The model under review builds one solid part; all positions refer to its coordinate system, in mm. Give positions to 0.01 mm unless a question says otherwise; leave off trailing zeros. Loops run counter-clockwise (first coordinate to the right, second up) from the corner with the lowest first, then second, coordinate; pieces in that order, holes last. Notation, with made-up numbers: (38.25, 88) - (88.25, 88) arc R11 cw to (88.25, 92) - close; hole circle Ø1 at (42.5, 48). An arc over 180 degrees is marked (long way). Answer as a JSON object with one key per item and string values.
from build123d import *

# Parameters (mm, degrees)
F0_R     = 2
F1_DEPTH = 9
F3_DEPTH = 9.001


with BuildPart() as f1:
    # F0 (on Front) → F1 (new body)
    with BuildSketch(Plane.XZ):
        Polygon((265.897079, -111.097285), (265.897079, 120.763555), (212.761675, 120.763555), (212.761675, 198.045397), (174.114259, 198.045397), (174.114259, 246.352586), (82.3411, 246.352586), (82.3411, 285.000002), (-130.196029, 285.000002), (-130.196029, 246.352586), (-217.152296, 246.352586), (-217.152296, 198.045397), (-265.461152, 198.045397), (-265.461152, 120.763555), (-182.215667, 120.657777), (-182.292131, 78.99439), (-40.622253, 80.756165), (-39.717878, 37.151925), (50.208882, 36.247385), (51.121586, -25.518982), (-39.717878, -26.429854), (-39.717878, -70.935305), (-180.510698, -71.846343), (-180.510698, -115.447249), (-265.897079, -116.364784), (-265.461152, -183.560564), (-217.152296, -183.560564), (-217.152296, -246.360741), (-130.196029, -246.360741), (-130.196029, -284.999998), (82.3411, -284.999998), (82.3411, -246.360741), (174.114259, -246.360741), (174.114259, -183.560564), (212.761675, -183.560564), (212.761675, -111.097285), align=None)
        with Locations((-169.174156, -241.860734)):
            Circle(F0_R, mode=Mode.SUBTRACT)
        with Locations((-236.821267, -179.060557)):
            Circle(F0_R, mode=Mode.SUBTRACT)
        with Locations((-212.652289, -210.460646)):
            Circle(F0_R, mode=Mode.SUBTRACT)
        with Locations((-261.179171, -149.93847)):
            Circle(F0_R, mode=Mode.SUBTRACT)
        with Locations((-125.696022, -261.180363)):
            Circle(F0_R, mode=Mode.SUBTRACT)
        with Locations((-23.927464, -280.499991)):
            Circle(F0_R, mode=Mode.SUBTRACT)
        with Locations((-218.689395, -120.357772)):
            Circle(F0_R, mode=Mode.SUBTRACT)
        with Locations((-176.010692, -98.108243)):
            Circle(F0_R, mode=Mode.SUBTRACT)
        with Locations((-105.614282, -75.861807)):
            Circle(F0_R, mode=Mode.SUBTRACT)
        with Locations((-35.217872, -53.145626)):
            Circle(F0_R, mode=Mode.SUBTRACT)
        with Locations((77.841094, -261.180363)):
            Circle(F0_R, mode=Mode.SUBTRACT)
        with Locations((123.727673, -241.860734)):
            Circle(F0_R, mode=Mode.SUBTRACT)
        with Locations((169.614252, -210.460646)):
            Circle(F0_R, mode=Mode.SUBTRACT)
        with Locations((188.937961, -179.060557)):
            Circle(F0_R, mode=Mode.SUBTRACT)
        with Locations((208.261669, -142.828918)):
            Circle(F0_R, mode=Mode.SUBTRACT)
        with Locations((10.235017, -30.429196)):
            Circle(F0_R, mode=Mode.SUBTRACT)
        with Locations((234.829371, -106.597278)):
            Circle(F0_R, mode=Mode.SUBTRACT)
        with Locations((-219.334275, 125.204953)):
            Circle(F0_R, mode=Mode.SUBTRACT)
        with Locations((-177.74558, 104.351434)):
            Circle(F0_R, mode=Mode.SUBTRACT)
        with Locations((-35.762538, 63.459567)):
            Circle(F0_R, mode=Mode.SUBTRACT)
        with Locations((-106.999755, 84.431064)):
            Circle(F0_R, mode=Mode.SUBTRACT)
        with Locations((-260.961145, 159.401619)):
            Circle(F0_R, mode=Mode.SUBTRACT)
        with Locations((-236.806717, 193.54539)):
            Circle(F0_R, mode=Mode.SUBTRACT)
        with Locations((-212.652289, 217.698985)):
            Circle(F0_R, mode=Mode.SUBTRACT)
        with Locations((-169.174156, 241.852579)):
            Circle(F0_R, mode=Mode.SUBTRACT)
        with Locations((-125.696022, 261.176288)):
            Circle(F0_R, mode=Mode.SUBTRACT)
        with Locations((-23.927464, 280.499996)):
            Circle(F0_R, mode=Mode.SUBTRACT)
        with Locations((55.165724, 5.364793)):
            Circle(F0_R, mode=Mode.SUBTRACT)
        with Locations((9.66711, 41.155414)):
            Circle(F0_R, mode=Mode.SUBTRACT)
        with Locations((261.397073, 4.833135)):
            Circle(F0_R, mode=Mode.SUBTRACT)
        with Locations((234.829371, 116.263548)):
            Circle(F0_R, mode=Mode.SUBTRACT)
        with Locations((123.727673, 241.852579)):
            Circle(F0_R, mode=Mode.SUBTRACT)
        with Locations((77.841094, 261.176288)):
            Circle(F0_R, mode=Mode.SUBTRACT)
        with Locations((188.937961, 193.54539)):
            Circle(F0_R, mode=Mode.SUBTRACT)
        with Locations((208.261669, 154.904469)):
            Circle(F0_R, mode=Mode.SUBTRACT)
        with Locations((169.614252, 217.698985)):
            Circle(F0_R, mode=Mode.SUBTRACT)
    extrude(amount=F1_DEPTH)

    # F2 (on face) → F3 (cut, through all)
    with BuildSketch(Plane(origin=(0, 0, 0), x_dir=(-1, 0, 0), z_dir=(0, 1, 0))):
        Polygon((-62.341114, 265.000015), (-62.341114, 226.352599), (-154.114272, 226.352599), (-154.114272, 178.04541), (-192.761689, 178.04541), (-192.761689, 100.763568), (-245.897092, 100.763568), (-245.897092, -91.097298), (-192.761689, -91.097298), (-192.761689, -163.560577), (-154.114272, -163.560577), (-154.114272, -226.360754), (-62.341114, -226.360754), (-62.341114, -265.000011), (110.196042, -265.000011), (110.196042, -226.360754), (197.152309, -226.360754), (197.152309, -163.560577), (245.590493, -163.560577), (245.768319, -136.149628), (160.510711, -135.233477), (160.510711, -91.717333), (19.717892, -90.806296), (19.717892, -46.230301), (-71.416299, -45.316474), (-69.918433, 56.050133), (20.124334, 56.95584), (21.037859, 101.001245), (162.254945, 99.245101), (162.178988, 140.63232), (245.461165, 140.738145), (245.461165, 178.04541), (197.152309, 178.04541), (197.152309, 226.352599), (110.196042, 226.352599), (110.196042, 265.000015), align=None)
    extrude(amount=-F3_DEPTH, mode=Mode.SUBTRACT)


solid = f1.part
Q1. To check wall thickness, follow probe 1 along X at (y, z) = (-6, 261.5); probe 2 along X at (y, z) = (-0.5, 166); probe 3 along X at (y, z) = (-1.75, -131). State the ranges of each line that lie inside material, in increasing order. Write a range as [from, to].
Results:
{"probe 1": "x = [-130.2, -127.67], [-123.72, -110.2], [62.34, 75.87], [79.81, 82.34]", "probe 2": "x = [-265.46, -245.46], [192.76, 212.76]", "probe 3": "x = [-265.8, -160.51], [192.76, 212.76]"}
Q2. Consider section A-A, the plane x = -79.5. State the section outline as (y, z) points.
Results:
{"outline": "(-9, -285) - (0, -285) - (0, -265) - (-9, -265) - close; (-9, -91.19) - (0, -91.19) - (0, -71.19) - (-9, -71.19) - close; (-9, 80.27) - (0, 80.27) - (0, 100.27) - (-9, 100.27) - close; (-9, 265) - (0, 265) - (0, 285) - (-9, 285) - close"}
Q3. Clearance check with flat-ended pins moving along their axes: pin 1 Ø4.5 at (x, y) = (-172.5, -5.5) entering from -Z; pin 2 Ø4.5 at (y, z) = (-6.5, 8.5) entering from -X; pin 3 Ø4.5 at (x, y) = (141.5, -4) entering from +Z; pin 4 Ø2.5 at (x, z) = (77.84, 261.18) entering from -Y. State where each tip first meets the part, or that it passes through.
Results:
{"pin 1": "stops at z = -246.36", "pin 2": "stops at x = 50.59", "pin 3": "stops at z = 246.35", "pin 4": "passes through"}
Q4. Consider section B-B, the plane y = -3.75. State how many separate pieces and enclosed holes the cut face has, plus the area to 3 significant figures.
Results:
{"separate pieces": "1", "enclosed holes": "37", "area": "54,600 mm^2"}
